Design review of the part built by this model. Coordinates are the model's own, in mm. A direction names the side the tool comes from. Coordinates: 2 decimals unless noted, no trailing zeros. Loops run counter-clockwise (first coordinate to the right, second up) from the corner with the lowest first, then second, coordinate; pieces in that order, holes last. Notation, with made-up numbers: M 70.25,31.25 L 87.25,31.25 A14 cw 87.25,50.25 Z; hole C 82,82.25 d7. An arc over 180 degrees is marked long. One line per item, written item: value.
```python
from build123d import *

# Parameters (mm, degrees)
F1_DEPTH = 32
F2_R     = 5.5
F3_DEPTH = 25
F4_R     = 6.5
F5_DEPTH = 113.001


with BuildPart() as f1:
    # F0 (on Front) → F1 (new body)
    with BuildSketch(Plane.XZ):
        Polygon((0, 13), (0, 0), (39, 0), (39, 17), (74, 17), (74, 0), (113, 0), (113, 13), (93, 13), (93, 64), (74, 64), (74, 30), (39, 30), (39, 64), (20, 64), (20, 13), align=None)
    extrude(amount=F1_DEPTH)

    # F2 (on Top) → F3 (cut)
    with BuildSketch(Plane.XY):
        with Locations((9.231269, -13)):
            Circle(F2_R)
        with Locations((103.805094, -13)):
            Circle(F2_R)
        Polygon((9.587883, 0), (0, 0), (0, -9.587883), align=None)
        Polygon((113, -9.757595), (113, 0), (103.242405, 0), align=None)
    extrude(amount=F3_DEPTH, mode=Mode.SUBTRACT)

    # F4 (on Right) → F5 (cut, through all)
    with BuildSketch(Plane.YZ):
        with Locations((-16, 46)):
            Circle(F4_R)
        with BuildLine():
            ThreePointArc((-32, 59.928225), (-16, 63.799461), (0, 59.928225))
            Line((0, 59.928225), (0, 64))
            Line((0, 64), (-32, 64))
            Line((-32, 64), (-32, 59.928225))
        make_face()
    extrude(amount=F5_DEPTH, mode=Mode.SUBTRACT)


solid = f1.part
```
(1) We need section B-B on y = -13. State how many separate pieces and enclosed holes the cut face has, then the cut area to 3 significant figures.
Reply:
separate pieces: 5
enclosed holes: 0
area: 2,670 mm2
(2) Mouldability with a two-part tool opening along X and no side actions: class faces 6 (the flat face through (113, -21, 6)), 7 (the flat face through (56, -16, 17)), 8 (the flat face through (10, -19, 13)) as released by +X, released by -X, zero draft, split by the parting line, or undercut.
Reply:
face 6: released by +X
face 7: undercut
face 8: zero draft
(3) Insertion check: pin 1 (8 mm diameter, centred on x = 60, y = -4.5, fed in from -Z); pin 2 (8 mm diameter, centred on y = -16, z = 46, fed in from -X); pin 3 (9.5 mm diameter, centred on y = -13, z = 38.5, fed in from +X); pin 4 (12.5 mm diameter, centred on x = 9.23, y = -13, fed in from +Z). Each pin has a flat end and moves straight along its axis. Give the tip position at first contact, or say it passes through.
Reply:
pin 1: stops at z = 17
pin 2: passes through
pin 3: stops at x = 93
pin 4: stops at z = 13
(4) We need section A-A on z = 46. State the section outline as (x, y) points.
Reply:
outline: M 20,-32 L 39,-32 L 39,-22.5 L 20,-22.5 Z; M 20,-9.5 L 39,-9.5 L 39,0 L 20,0 Z; M 74,-32 L 93,-32 L 93,-22.5 L 74,-22.5 Z; M 74,-9.5 L 93,-9.5 L 93,0 L 74,0 Z
(5) To check wall thickness, follow line 1 along X through (y, z) = (-13, 7); line 2 along X through (y, z) = (-11.5, 56); line 3 along Y through (x, z) = (83, 46). State the ranges of each line that lie inside material, in increasing order. Write a range as [from, to].
Reply:
line 1: x = [0, 3.73], [14.73, 39], [74, 98.31], [109.31, 113]
line 2: x = [20, 39], [74, 93]
line 3: y = [-32, -22.5], [-9.5, 0]
(6) Tool access review of faces 1 (the flat face through (39, -16, 8)), 2 (the flat face through (74, -23, 47)), 3 (the flat face through (20, -16, 39)), 4 (the flat face through (93, -16, 38)), 5 (the flat face through (19, -16, 0)): name each direction out of +Z, -Z, +X, -X, +Y, -Y from which nothing blocks a thin tool from reaching the whole face with its end or side.
Reply:
face 1: -Z, +Y, -Y
face 2: +Z, +Y, -Y
face 3: +Z, -X, +Y, -Y
face 4: +Z, +X, +Y, -Y
face 5: -Z, +X, -X, +Y, -Y
(7) We need section C-C on x = 80. State the section outline as (y, z) points.
Reply:
outline: M -32,0 L 0,0 L 0,59.93 A35 ccw -32,59.93 Z; hole C -16,46 d13
(8) We need section D-D on y = -3. State the section outline as (x, z) points.
Reply:
outline: M 6.59,0 L 39,0 L 39,17 L 74,17 L 74,0 L 106.24,0 L 106.24,13 L 93,13 L 93,61.3 L 74,61.3 L 74,30 L 39,30 L 39,61.3 L 20,61.3 L 20,13 L 6.59,13 Z
